Here's the drawing with two shaded views (mm, measured from the low corner). I have some questions. A direction names the side the tool comes from. Give positions to 0.01 mm unless a question says otherwise; leave off trailing zeros. Write each loop counter-clockwise with the first axis right and the second up, starting at its lowest first coordinate (ties: lowest second). Pieces come first, ordered by that corner, then holes. Notation, with made-up numbers: M 25.5,-2 L 57.5,-2 A29 cw 57.5,34 Z; hole C -21.75,11.25 d9. An arc over 180 degrees is marked long. Answer as a JSON object with one key per item and string values. Group by question number.
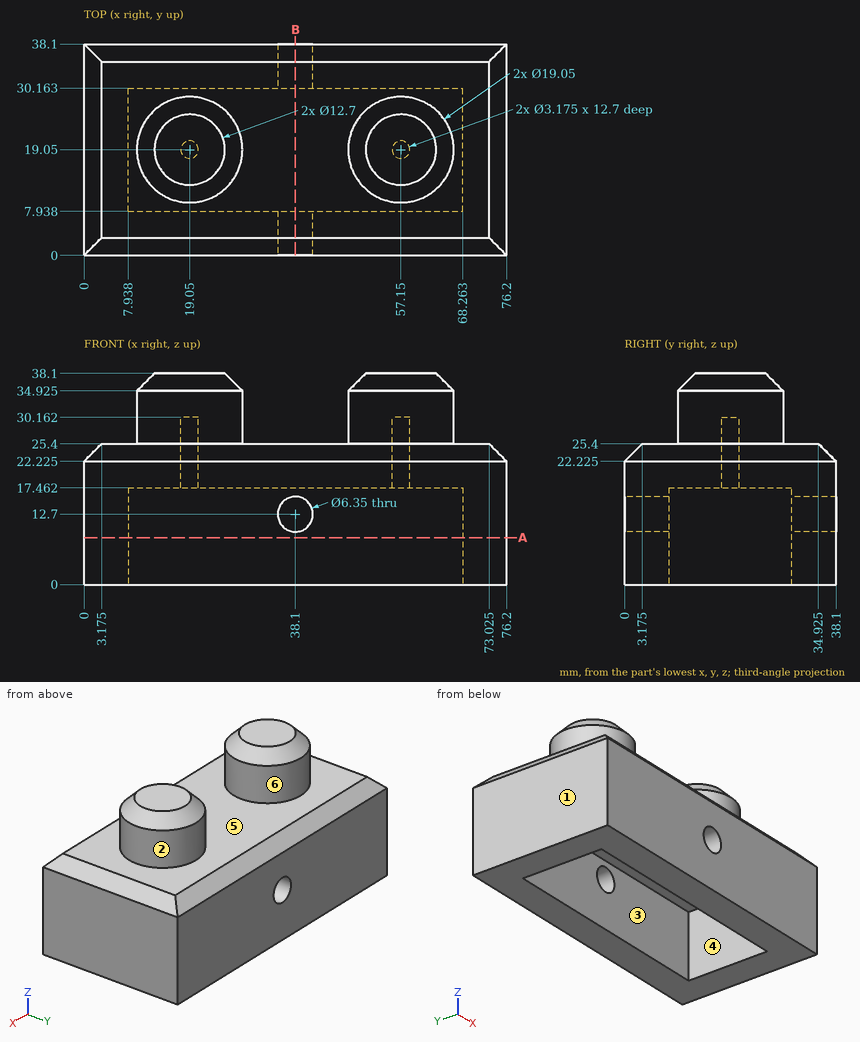
1) For the marked faces 1 and 2, which set-ups out of +Z, -Z, +X, -X, +Y, -Y let a thin tool reach every point of the face, with its end or its side?
2) If we section it at B-B, the plane x = 38.1: List the corners of the cut face in (y, z) for me (1 decimal).
3) We'd pull the mould along Y, two halves only. Please class the marked faces 3, 4, 5 and 6: released by +Y, released by -Y, zero draft, split by the parting line, or undercut.
4) If we section it at A-A, the plane z = 8.5: List the corners of the cut face in (x, y) for me.
5) Please list where these lines run through material, in increasing order: line 1 along X through (y, z) = (19, 20); line 2 along X through (y, z) = (27, 4); line 3 along Y through (x, z) = (50, 15.5). Write a range as from..to.
6) I'm going to push flat-ended pins straight in: pin 1 (1 mm diameter, centred on x = 15.5, y = 13.5, fed in from -Z); pin 2 (19 mm diameter, centred on x = 48.5, z = 9.5, fed in from -Y); pin 3 (1 mm diameter, centred on x = 19.5, y = 19, fed in from -Z); pin 4 (4 mm diameter, centred on x = 12, z = 24.5, fed in from -Y) (1 decimal). Where does each tip first touch, or does it pass through?
Taken from the geometry:
{
 "1": {"face 1": "+Z, -Z, -X, +Y, -Y", "face 2": "+Z"},
 "2": {"outline": "M 0,0 L 7.9,0 L 7.9,9.5 L 0,9.5 Z; M 0,15.9 L 7.9,15.9 L 7.9,17.5 L 30.2,17.5 L 30.2,15.9 L 38.1,15.9 L 38.1,22.2 L 34.9,25.4 L 3.2,25.4 L 0,22.2 Z; M 30.2,0 L 38.1,0 L 38.1,9.5 L 30.2,9.5 Z"},
 "3": {"face 3": "undercut", "face 4": "undercut", "face 5": "zero draft", "face 6": "split by the parting line"},
 "4": {"outline": "M 0,0 L 76.2,0 L 76.2,38.1 L 0,38.1 Z; hole M 7.94,7.94 L 68.26,7.94 L 68.26,30.16 L 7.94,30.16 Z"},
 "5": {"line 1": "0..17.46, 20.64..55.56, 58.74..76.2", "line 2": "0..7.94, 68.26..76.2", "line 3": "0..7.94, 30.16..38.1"},
 "6": {"pin 1": "z = 17.46", "pin 2": "y = 0", "pin 3": "z = 30.16", "pin 4": "y = 0.3"}
}
